Read the model definition and answer for the solid it produces. Units are mm, in the model's axes. Round coordinates to 2 decimals unless told otherwise and drop trailing zeros. Write each loop counter-clockwise with the first axis right and the second up, starting at its lowest first coordinate (ties: lowest second). Pieces come first, ordered by that corner, then holes. Notation, with made-up numbers: (54, -21.5) - (107, -21.5) arc R24 cw to (107, 3.5) - close; hole circle Ø9 at (49, 62). An arc over 180 degrees is marked (long way). Answer as CSV lines item,"result". Start each with the question number.
1) Find section C-C on y = -4.1. Determine the outline of the cut face in (x, z) (3 decimals), then the cut area to 3 significant figures.
2) Find section B-B on x = 0. Determine the outline of the cut face in (y, z) (1 decimal), then the cut area to 3 significant figures.
3) Find section A-A on z = 0. Determine the outline of the cut face in (x, y) (1 decimal), then the cut area to 3 significant figures.
4) Each of these flat-tipped pins is pushed along its axis until it touches: pin 1 (1.8 mm diameter, centred on x = 21.875, z = -6.525, fed in from +Y); pin 2 (2.5 mm diameter, centred on x = -8.475, z = -6.525, fed in from +Y) (3 decimals). Where does it stop, or does it pass through?
5) Consider line 1 along X through (y, z) = (-3.95, -6.5); line 2 along X through (y, z) = (-3.75, 5); line 3 along Z through (x, y) = (-5.5, -4.2) (3 decimals). Determine where each line is inside the solid, lowest interval first.
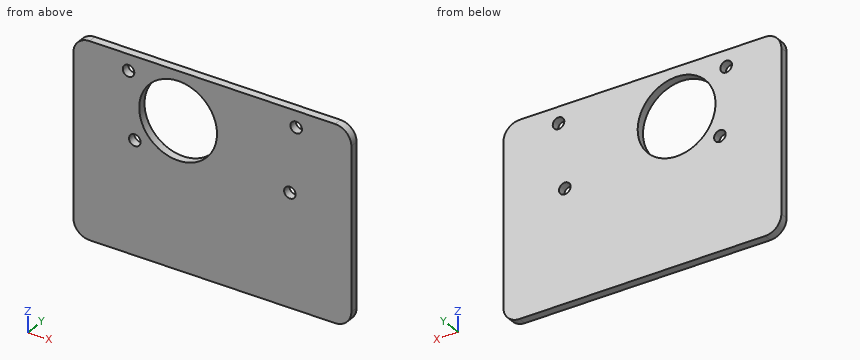
from build123d import *

# Parameters (mm, degrees)
SKETCH_1_R      = 7.62
SKETCH_1_R_2    = 1.1303
EXTRUDE_1_DEPTH = 1.5875


with BuildPart() as part:
    # 草图1 → 凸台-拉伸1 (new body)
    with BuildSketch(Plane.XZ.offset(4.7625)):
        with BuildLine():
            Line((33.9, -25.4), (33.9, 6.35))
            ThreePointArc((33.9, 6.35), (32.97006403, 8.59506403), (30.725, 9.525))
            Line((30.725, 9.525), (-17.325, 9.525))
            ThreePointArc((-17.325, 9.525), (-19.57006403, 8.59506403), (-20.5, 6.35))
            Line((-20.5, 6.35), (-20.5, -25.4))
            ThreePointArc((-20.5, -25.4), (-19.57006403, -27.64506403), (-17.325, -28.575))
            Line((-17.325, -28.575), (30.725, -28.575))
            ThreePointArc((30.725, -28.575), (32.97006403, -27.64506403), (33.9, -25.4))
        make_face()
        Circle(SKETCH_1_R, mode=Mode.SUBTRACT)
        with Locations((-9.705, 6.35)):
            Circle(SKETCH_1_R_2, mode=Mode.SUBTRACT)
        with Locations((23.105, 6.35)):
            Circle(SKETCH_1_R_2, mode=Mode.SUBTRACT)
        with Locations((21.875, -6.525)):
            Circle(SKETCH_1_R_2, mode=Mode.SUBTRACT)
        with Locations((-8.475, -6.525)):
            Circle(SKETCH_1_R_2, mode=Mode.SUBTRACT)
    extrude(amount=-EXTRUDE_1_DEPTH)


solid = part.part
Check values:
1,outline,"(-20.5, -25.4) arc R3.175 ccw to (-17.325, -28.575) - (30.725, -28.575) arc R3.175 ccw to (33.9, -25.4) - (33.9, 6.35) arc R3.175 ccw to (30.725, 9.525) - (-17.325, 9.525) arc R3.175 ccw to (-20.5, 6.35) - close; hole circle Ø2.261 at (-9.705, 6.35); hole circle Ø2.261 at (-8.475, -6.525); hole circle Ø15.24 at (0, 0); hole circle Ø2.261 at (21.875, -6.525); hole circle Ø2.261 at (23.105, 6.35)"
1,area,"1,870 mm^2"
2,outline,"(-4.8, -28.6) - (-3.2, -28.6) - (-3.2, -7.6) - (-4.8, -7.6) - close; (-4.8, 7.6) - (-3.2, 7.6) - (-3.2, 9.5) - (-4.8, 9.5) - close"
2,area,"36.3 mm^2"
3,outline,"(-20.5, -4.8) - (-7.6, -4.8) - (-7.6, -3.2) - (-20.5, -3.2) - close; (7.6, -4.8) - (33.9, -4.8) - (33.9, -3.2) - (7.6, -3.2) - close"
3,area,"62.2 mm^2"
4,pin 1,"passes through"
4,pin 2,"stops at y = -3.175"
5,line 1,"x = -20.5 to -9.61, -7.34 to -3.98, 3.98 to 20.74, 23.01 to 33.9"
5,line 2,"x = -20.5 to -5.75, 5.75 to 33.9"
5,line 3,"z = -28.575 to -5.274, 5.274 to 9.525"
